Source: CAD feature listing. Evaluate the final solid. Frame: model axes, mm. Face numbers are marked on the shaded views. A direction names the side the tool comes from. Round coordinates to 2 decimals unless told otherwise and drop trailing zeros. Loops run counter-clockwise (first coordinate to the right, second up) from the corner with the lowest first, then second, coordinate; pieces in that order, holes last.
(1) Set-up query: the marked faces 1, 2 and 3. Return all of +Z, -Z, +X, -X, +Y, -Y with unobstructed straight access to the full face (end or side cutting, diameter ignored); none if empty.
(2) Section A-A, the plane x = -61. Return the cut outline in (y, z).
(3) Material intervals for probe 1 along Y at (x, z) = (7, 8); probe 2 along Y at (x, z) = (-89, 5); probe 3 along Z at (x, y) = (9, 80.5), sorted ascending.
(4) First-contact query: pin 1 Ø4 at (x, y) = (-87.5, 17.5) entering from +Z; pin 2 Ø8 at (x, y) = (-91.54, 91.29) entering from -Z; pin 3 Ø5.5 at (x, y) = (7.06, 91.29) entering from -Z; pin 4 Ø14.5 at (x, y) = (-22, 11) entering from +Z. Flat tips, straight axial feed; report the tip coordinate or a pass-through.
(5) Section C-C, the plane y = -31.5. Return the cut outline in (x, z), plus the area to 3 significant figures.
(6) Section B-B, the plane z = 9.5. Return the cut outline in (x, y).
(7) Section D-D, the plane x = -37. Return the cut outline in (y, z), plus the area to 3 significant figures.
```python
from build123d import *

# Parameters (mm, degrees)
F1_DEPTH = 25
F2_R     = 3
F3_DEPTH = 1000
F4_R     = 14.543021
F5_DEPTH = 6.5
F6_R     = 9
F7_DEPTH = 5.4


with BuildPart() as f1:
    # F0 (on Top) → F1 (new body)
    with BuildSketch(Plane.XY):
        Polygon((16.063117, -18.205635), (16.063117, 100.294365), (-100.53736, 100.294365), (-100.53736, -48.205635), (-51.03736, -48.205635), (-51.03736, -18.205635), align=None)
    extrude(amount=F1_DEPTH)

    # F2 (on face) → F3 (cut)
    with BuildSketch(Plane.XY.offset(25)):
        with Locations((7.063117, 91.294365)):
            Circle(F2_R)
        with Locations((7.063117, -9.286914)):
            Circle(F2_R)
        with Locations((-91.53736, 91.294365)):
            Circle(F2_R)
        with Locations((-91.53736, -9.286914)):
            Circle(F2_R)
    extrude(amount=-F3_DEPTH, mode=Mode.SUBTRACT)

    # F4 (on face) → F5 (join)
    with BuildSketch(Plane.XY.offset(25)):
        with Locations((-64.53736, 13.794365)):
            Circle(F4_R)
    extrude(amount=F5_DEPTH)

    # F6 (on face) → F7 (join)
    with BuildSketch(Plane.XY.offset(25)):
        with Locations((-0.03736, 13.794365)):
            Circle(F6_R)
        with Locations((-25.53736, 13.794365)):
            Circle(F6_R)
    extrude(amount=F7_DEPTH)


solid = f1.part
```
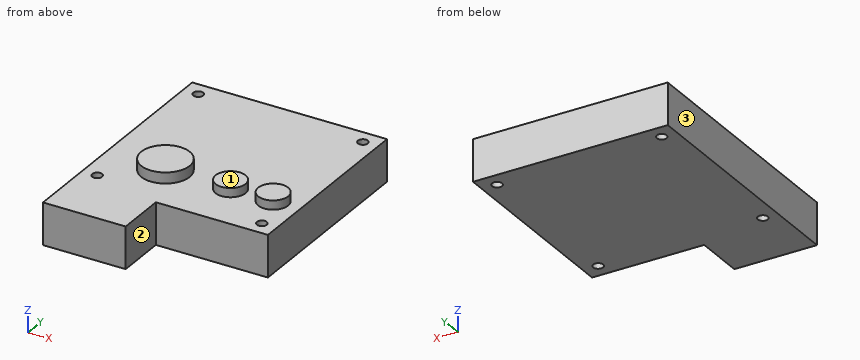
Output values:
1. face 1: +Z, +X, +Y, -Y
1. face 2: +Z, -Z, +X, -Y
1. face 3: +Z, -Z, -X, +Y, -Y
2. outline: (-48.21, 0) - (100.29, 0) - (100.29, 25) - (27.9, 25) - (27.9, 31.5) - (-0.31, 31.5) - (-0.31, 25) - (-48.21, 25) - close
3. probe 1: y = -18.21 to -12.29, -6.29 to 88.3, 94.29 to 100.29
3. probe 2: y = -48.21 to -10.89, -7.69 to 89.69, 92.89 to 100.29
3. probe 3: z = 0 to 25
4. pin 1: stops at z = 25
4. pin 2: stops at z = 0
4. pin 3: passes through
4. pin 4: stops at z = 30.4
5. outline: (-100.54, 0) - (-51.04, 0) - (-51.04, 25) - (-100.54, 25) - close
5. area: 1,240 mm2
6. outline: (-100.54, -48.21) - (-51.04, -48.21) - (-51.04, -18.21) - (16.06, -18.21) - (16.06, 100.29) - (-100.54, 100.29) - close; hole circle Ø6 at (-91.54, -9.29); hole circle Ø6 at (-91.54, 91.29); hole circle Ø6 at (7.06, -9.29); hole circle Ø6 at (7.06, 91.29)
7. outline: (-18.21, 0) - (100.29, 0) - (100.29, 25) - (-18.21, 25) - close
7. area: 2,960 mm2
